Check sheet for the modelled part. Datum: model origin and axes. Units: mm. Face numbers are marked on the shaded views. A direction names the side the tool comes from. Give positions to 0.01 mm unless a question says otherwise; leave off trailing zeros. Write each loop counter-clockwise with the first axis right and the second up, starting at its lowest first coordinate (ties: lowest second). Pieces come first, ordered by that corner, then holes. Notation, with made-up numbers: (44.5, -6) -> (66.5, -6) arc R12 cw to (66.5, 7) -> close; hole circle Ø1 at (71, -32.5). An arc over 180 degrees is marked (long way). Answer as a JSON object with one key per item and string values.
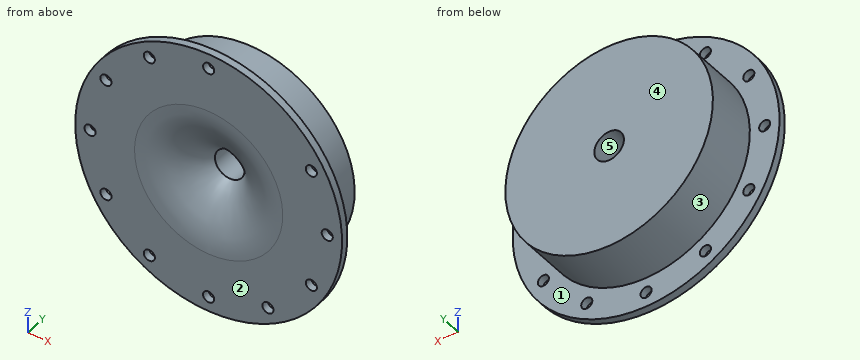
from build123d import *

# Parameters (mm, degrees)
F_3_8_0_375_DIAMETER_HOLE2_D = 9.525
CIRPATTERN2_COUNT            = 12


with BuildPart() as part:
    # Sketch1 → Revolve1 (revolve)
    with BuildSketch(Plane.XY, mode=Mode.PRIVATE) as revolve1_sk:
        with BuildLine():
            Line((12.7, 50.8), (12.7, 25.4))
            ThreePointArc((12.7, 25.4), (35.101936686, 6.703873372), (63.5, 0))
            Line((63.5, 0), (114.3, 0))
            Line((114.3, 0), (114.3, 6.35))
            Line((114.3, 6.35), (88.9, 6.35))
            Line((88.9, 6.35), (88.9, 50.8))
            Line((88.9, 50.8), (12.7, 50.8))
        make_face()
    revolve(revolve1_sk.sketch.rotate(Axis((0, 0, 0), (0, 1, 0)), 90), axis=Axis((0, 0, 0), (0, 1, 0)))

    # 3/8 (0.375) Diameter Hole2 (through all)
    with Locations(Plane(origin=(0, 6.35, 0), x_dir=(1, 0, 0), z_dir=(0, 1, 0))):
        with Locations((0, -101.6)):
            f_3_8_0_375_diameter_hole2 = Hole(F_3_8_0_375_DIAMETER_HOLE2_D / 2)

    # CirPattern2: 3/8 (0.375) Diameter Hole2 ×12 about axis, 1 skipped
    cirpattern2_axis = Axis((0, 0, 0), (0, 1, 0))
    add([f_3_8_0_375_diameter_hole2.rotate(cirpattern2_axis, i * 360 / CIRPATTERN2_COUNT) for i in range(1, CIRPATTERN2_COUNT) if i not in (1,)], mode=Mode.SUBTRACT)


solid = part.part
1. Go/stop test with flat-tipped pins: P1, Ø5.5, axis at x = 87.99, z = -50.8, coming from the +Y side; P2, Ø2, axis at y = 29.5, z = 17.5, coming from the +X side; P3, Ø5, axis at x = 24, y = 10.5, coming from the +Z side; P4, Ø15, axis at x = 0, z = -101.6, coming from the +Y side. Record where each tip stops, or that it passes through.
Determined:
{"P1": "through", "P2": "x = 87.36", "P3": "z = 86.26", "P4": "y = 6.35"}
2. Scan lines: L1, parallel to Y at x = 88.5, z = 24.5; L2, parallel to X at y = 4, z = 101.6; L3, parallel to Z at x = 4, y = 34.5. Record each from-to range of solid material in increasing order. Write a range as [from, to].
Determined:
{"L1": "[0, 6.35]", "L2": "[-52.36, -4.76], [4.76, 52.36]", "L3": "[-88.81, -12.05], [12.05, 88.81]"}
3. Mould release check, pull along X, two halves, no side actions. Record for the marked faces 3, 4 and 5: released by +X, released by -X, zero draft, split by the parting line, or undercut.
Determined:
{"face 3": "split by the parting line", "face 4": "zero draft", "face 5": "undercut"}
4. Sectioned sample at A-A, the plane z = -101.6. Enter the section's corners in (x, y).
Determined:
{"outline": "(-52.36, 0) -> (-4.76, 0) -> (-4.76, 6.35) -> (-52.36, 6.35) -> close; (4.76, 0) -> (52.36, 0) -> (52.36, 6.35) -> (4.76, 6.35) -> close"}
5. Sectioned sample at D-D, the plane z = 75. Enter the section's corners in (x, y), plus the area to 3 significant figures.
Determined:
{"outline": "(-86.25, 0) -> (86.25, 0) -> (86.25, 6.35) -> (47.73, 6.35) -> (47.73, 50.8) -> (-47.73, 50.8) -> (-47.73, 6.35) -> (-86.25, 6.35) -> close", "area": "5,340 mm^2"}
6. Access from +Z, -Z, +X, -X, +Y, -Y to the whole of each face (thin tool, end or side, straight path). Record for the marked faces 1 and 2.
Determined:
{"face 1": "+Y", "face 2": "+Z, -Z, +X, -X, -Y"}
7. Sectioned sample at B-B, the plane y = 32.5. Enter the section's corners in (x, z), plus the area to 3 significant figures.
Determined:
{"outline": "circle Ø177.8 at (0, 0); hole circle Ø25.4 at (0, 0)", "area": "24,300 mm^2"}
8. Sectioned sample at C-C, the plane x = -101.6. Enter the section's corners in (y, z), plus the area to 3 significant figures.
Determined:
{"outline": "(0, -52.36) -> (6.35, -52.36) -> (6.35, -4.76) -> (0, -4.76) -> close; (0, 4.76) -> (6.35, 4.76) -> (6.35, 52.36) -> (0, 52.36) -> close", "area": "605 mm^2"}
